Here's how the part is built. I have some questions about the finished solid (model axes, mm). Coordinates: 2 decimals unless noted, no trailing zeros. Write each loop counter-clockwise with the first axis right and the second up, starting at its lowest first coordinate (ties: lowest second). Pieces come first, ordered by that corner, then holes. Notation, with made-up numbers: M 43,-14 L 99,-14 A17 ccw 99,-4 Z; hole C 47,69.5 d7. An arc over 180 degrees is marked long. Use a Markdown table: item, result.
```python
from build123d import *

# Parameters (mm, degrees)
ESQUISSE2_R        = 32
ESQUISSE2_R_2      = 30
BOSS_EXTRU_2_DEPTH = 60
ESQUISSE3_R        = 32
BOSS_EXTRU_3_DEPTH = 1
CONG_1_R           = 10


with BuildPart() as part:
    # Esquisse2 → Boss.-Extru.2 (new body)
    with BuildSketch(Plane(origin=(0, 0, 0), x_dir=(1, 0, 0), z_dir=(0, 1, 0))):
        with Locations(Location((0, 0, 0), (0, 0, 270))):
            Circle(ESQUISSE2_R)
        with Locations(Location((0, 0, 0), (0, 0, 270))):
            Circle(ESQUISSE2_R_2, mode=Mode.SUBTRACT)
    extrude(amount=BOSS_EXTRU_2_DEPTH)

    # Esquisse3 → Boss.-Extru.3 (add)
    with BuildSketch(Plane.XZ):
        with Locations(Location((0, 0, 0), (0, 0, 90))):
            Circle(ESQUISSE3_R)
    extrude(amount=-BOSS_EXTRU_3_DEPTH)

    # Congé1
    cong_1_edges = [part.edges().sort_by_distance(p)[0] for p in [
        (0, 1, -30),
    ]]
    fillet(cong_1_edges, radius=CONG_1_R)


solid = part.part
```
1. Will these pins go through, and if not, where does the flat tip stop? pin 1 Ø3 at (y, z) = (37, 18) entering from -X; pin 2 Ø1 at (x, z) = (-23, 25) entering from -Y; pin 3 Ø5 at (y, z) = (25, -24) entering from -X; pin 4 Ø5 at (x, y) = (-4, 16.5) entering from -Z.
Answers follow:
| item | result |
|---|---|
| pin 1 | stops at x = -27.42 |
| pin 2 | passes through |
| pin 3 | stops at x = -23.7 |
| pin 4 | stops at z = -31.96 |
2. Suppose I cut it at A-A on z = 0. Write out the boundary of the cut face in (x, y).
Answers follow:
| item | result |
|---|---|
| outline | M -32,0 L 32,0 L 32,60 L 30,60 L 30,11 A10 cw 20,1 L -20,1 A10 cw -30,11 L -30,60 L -32,60 Z |
3. Suppose I cut it at C-C on y = 19. Write out the boundary of the cut face in (x, z), and give its area (3 significant figures).
Answers follow:
| item | result |
|---|---|
| outline | C 0,0 d64; hole C 0,0 d60 |
| area | 390 mm2 |
4. Suppose I cut it at B-B on x = 0. Write out the boundary of the cut face in (y, z).
Answers follow:
| item | result |
|---|---|
| outline | M 0,-32 L 60,-32 L 60,-30 L 11,-30 A10 cw 1,-20 L 1,20 A10 cw 11,30 L 60,30 L 60,32 L 0,32 Z |
5. I need wall thicknesses on probe 1 along X at (y, z) = (38, 0); probe 2 along X at (y, z) = (26.5, -12.5). Which ranges of each line are inside material? Lowest first, please.
Answers follow:
| item | result |
|---|---|
| probe 1 | x = -32 to -30, 30 to 32 |
| probe 2 | x = -29.46 to -27.27, 27.27 to 29.46 |
6. We'd pull the mould along X, two halves only. Please class faces 1 (the face through (0, 1, 0)), 2 (the face through (-31.24, 29.58, -6.94)), 3 (the face through (1.32, 35.16, -29.97)), 4 (the face through (0, 0, 0)): +X half, -X half, draft (parallel to the pull), parting line (faces both ways), or undercut.
Answers follow:
| item | result |
|---|---|
| face 1 | undercut |
| face 2 | parting line |
| face 3 | undercut |
| face 4 | draft |
